Could you check a few things on this model? Use its own coordinates, in mm. Face numbers are marked on the shaded views. A direction names the side the tool comes from. Round coordinates to 2 decimals unless told otherwise and drop trailing zeros. Order: outer loops, then holes, each group sorted by start corner. A loop starts at its lowest first (then second) coordinate and runs counter-clockwise, first axis right, second up. Notation, with made-up numbers: M -10.5,81.5 L 9.5,81.5 A25 ccw 9.5,113.5 Z; hole C -1,50 d2. An arc over 180 degrees is marked long. Write each question's results on one line, items separated by ' | '. Start each with the question number.
1. I'm going to push flat-ended pins straight in: pin 1 (0.8 mm diameter, centred on x = 7.5, z = 0.5, fed in from +Y); pin 2 (2.5 mm diameter, centred on x = -16.22, z = -11, fed in from +Y). Where does each tip first touch, or does it pass through?
2. Suppose I cut it at A-A on x = 9. Write out the boundary of the cut face in (y, z), and give its area (3 significant figures).
3. Suppose I cut it at C-C on y = -11. Write out the boundary of the cut face in (x, z), and give its area (3 significant figures).
4. Please list where these lines run through material, in increasing order: L1, parallel to Z at x = -14.4, y = -13.2; L2, parallel to Z at x = -13, y = -4.75; L3, parallel to Y at x = -16.2, z = -22.65.
5. For the marked faces 1 and 2, which set-ups out of +Z, -Z, +X, -X, +Y, -Y let a thin tool reach every point of the face, with its end or its side?
6. We'd pull the mould along Z, two halves only. Please class the marked faces 3, 4 and 5: released by +Z, released by -Z, zero draft, split by the parting line, or undercut.
7. Suppose I cut it at B-B on z = -15.4. Write out the boundary of the cut face in (x, y), and give its area (3 significant figures).
8. Suppose I cut it at D-D on y = -1.75. Write out the boundary of the cut face in (x, z), and give its area (3 significant figures).
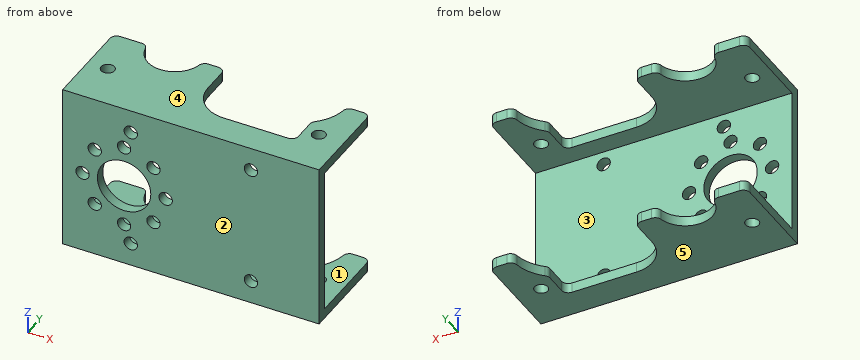
from build123d import *

# Parameters (mm, degrees)
F0_W     = 38.4
F0_H     = 28.4
F0_R     = 1
F0_R_2   = 4.1
F1_DEPTH = 1.5
F2_W     = 38.4
F2_H     = 1.5
F3_DEPTH = 22
F6_W     = 38.4
F6_H     = 14.2
F7_DEPTH = 25.001
F8_R     = 1
F8_R_2   = 4
F9_DEPTH = 1.5
F10_R    = 1


with BuildPart() as f1:
    # F0 (on Top) → F1 (new body)
    with BuildSketch(Plane.XY):
        Rectangle(F0_W, F0_H)
        with Locations((-16.2, -7.2)):
            Circle(F0_R, mode=Mode.SUBTRACT)
        with Locations((15.4, -7.2)):
            Circle(F0_R, mode=Mode.SUBTRACT)
        with Locations((-10, 0)):
            Circle(F0_R_2, mode=Mode.SUBTRACT)
        with Locations((-16.2, 7.2)):
            Circle(F0_R, mode=Mode.SUBTRACT)
        with BuildLine():
            ThreePointArc((-2.5, 4.8), (-1.0355339059, 8.3355339059), (2.5, 9.8))
            Line((2.5, 9.8), (12.2, 9.8))
            ThreePointArc((12.2, 9.8), (12.9071067812, 9.5071067812), (13.2, 8.8))
            Line((13.2, 8.8), (13.2, 5.5901699437))
            ThreePointArc((13.2, 5.5901699437), (13.2871290708, 5.1819216533), (13.5333333333, 4.8448139512))
            ThreePointArc((13.5333333333, 4.8448139512), (15.7, 0), (13.5333333333, -4.8448139512))
            ThreePointArc((13.5333333333, -4.8448139512), (13.2871290708, -5.1819216533), (13.2, -5.5901699437))
            Line((13.2, -5.5901699437), (13.2, -8.8))
            ThreePointArc((13.2, -8.8), (12.9071067812, -9.5071067812), (12.2, -9.8))
            Line((12.2, -9.8), (2.5, -9.8))
            ThreePointArc((2.5, -9.8), (-1.0355339059, -8.3355339059), (-2.5, -4.8))
            Line((-2.5, -4.8), (-2.5, 4.8))
        make_face(mode=Mode.SUBTRACT)
        with Locations((15.4, 7.2)):
            Circle(F0_R, mode=Mode.SUBTRACT)
    extrude(amount=F1_DEPTH)

    # F2 (on face) → F3 (join)
    with BuildSketch(Plane(origin=(0, 0, 0), x_dir=(1, 0, 0), z_dir=(0, 0, -1))):
        with Locations((0, 13.45)):
            Rectangle(F2_W, F2_H)
    extrude(amount=F3_DEPTH)

    # F5: F1 across plane


with BuildPart() as f1_1:
    add(f1.part)
    add(f1.part.mirror(Plane.XY.offset(-11)))

    # F6 (on face) → F7 (cut, through all)
    with BuildSketch(Plane(origin=(0, 0, -23.5), x_dir=(1, 0, 0), z_dir=(0, 0, -1))):
        with Locations((0, -7.1)):
            Rectangle(F6_W, F6_H)
    extrude(amount=-F7_DEPTH, mode=Mode.SUBTRACT)

    # F8 (on face) → F9 (cut, through all)
    with BuildSketch(Plane.XZ.offset(14.2)):
        with Locations((9, -2)):
            Circle(F8_R)
        with Locations((-9, -2)):
            Circle(F8_R)
        with Locations((-9, -20)):
            Circle(F8_R)
        with Locations((9, -20)):
            Circle(F8_R)
        with Locations((-10, -11)):
            Circle(F8_R_2)
        with Locations((-5.6, -6.6)):
            Circle(F8_R)
        with Locations((-10, -4.7774603256)):
            Circle(F8_R)
        with Locations((-14.4, -6.6)):
            Circle(F8_R)
        with Locations((-16.2225396744, -11)):
            Circle(F8_R)
        with Locations((-14.4, -15.4)):
            Circle(F8_R)
        with Locations((-10, -17.2225396744)):
            Circle(F8_R)
        with Locations((-5.6, -15.4)):
            Circle(F8_R)
        with Locations((-3.7774603256, -11)):
            Circle(F8_R)
    extrude(amount=-F9_DEPTH, mode=Mode.SUBTRACT)

    # F10
    f10_edges = [f1_1.edges().sort_by_distance(p)[0] for p in [
        (-19.2, 0, -22.75),
        (-19.2, 0, 0.75),
        (-5.9, 0, 0.75),
        (-14.1, 0, 0.75),
        (-5.9, 0, -22.75),
        (-14.1, 0, -22.75),
        (-2.5, 0, -22.75),
        (15.7, 0, -22.75),
        (15.7, 0, 0.75),
        (19.2, 0, -22.75),
        (19.2, 0, 0.75),
        (-2.5, 0, 0.75),
    ]]
    fillet(f10_edges, radius=F10_R)


solid = f1_1.part
Filled sheet:
1) pin 1: stops at y = -9.8 | pin 2: stops at y = -12.7
2) outline: M -14.2,-23.5 L -9.8,-23.5 L -9.8,-22 L -12.7,-22 L -12.7,-21 L -14.2,-21 Z; M -14.2,-19 L -12.7,-19 L -12.7,-3 L -14.2,-3 Z; M -14.2,-1 L -12.7,-1 L -12.7,0 L -9.8,0 L -9.8,1.5 L -14.2,1.5 Z | area: 40.2 mm^2
3) outline: M -19.2,-23.5 L 19.2,-23.5 L 19.2,-22 L -19.2,-22 Z; M -19.2,0 L 19.2,0 L 19.2,1.5 L -19.2,1.5 Z | area: 115 mm^2
4) L1: z = -23.5 to -16.4, -14.4 to -7.6, -5.6 to 1.5 | L2: z = -23.5 to -22, 0 to 1.5 | L3: y = -14.2 to -8.2, -6.2 to 0
5) face 1: +X, -X, +Y | face 2: +Z, -Z, +X, -X, -Y
6) face 3: undercut | face 4: released by +Z | face 5: released by -Z
7) outline: M -19.2,-14.2 L -15.4,-14.2 L -15.4,-12.7 L -19.2,-12.7 Z; M -13.4,-14.2 L -6.6,-14.2 L -6.6,-12.7 L -13.4,-12.7 Z; M -4.6,-14.2 L 19.2,-14.2 L 19.2,-12.7 L -4.6,-12.7 Z | area: 51.6 mm^2
8) outline: M -19.2,-23.5 L -13.71,-23.5 L -13.71,-22 L -19.2,-22 Z; M -19.2,0 L -13.71,0 L -13.71,1.5 L -19.2,1.5 Z; M -6.29,-23.5 L -2.5,-23.5 L -2.5,-22 L -6.29,-22 Z; M -6.29,0 L -2.5,0 L -2.5,1.5 L -6.29,1.5 Z; M 15.46,-23.5 L 19.2,-23.5 L 19.2,-22 L 15.46,-22 Z; M 15.46,0 L 19.2,0 L 19.2,1.5 L 15.46,1.5 Z | area: 39.1 mm^2
